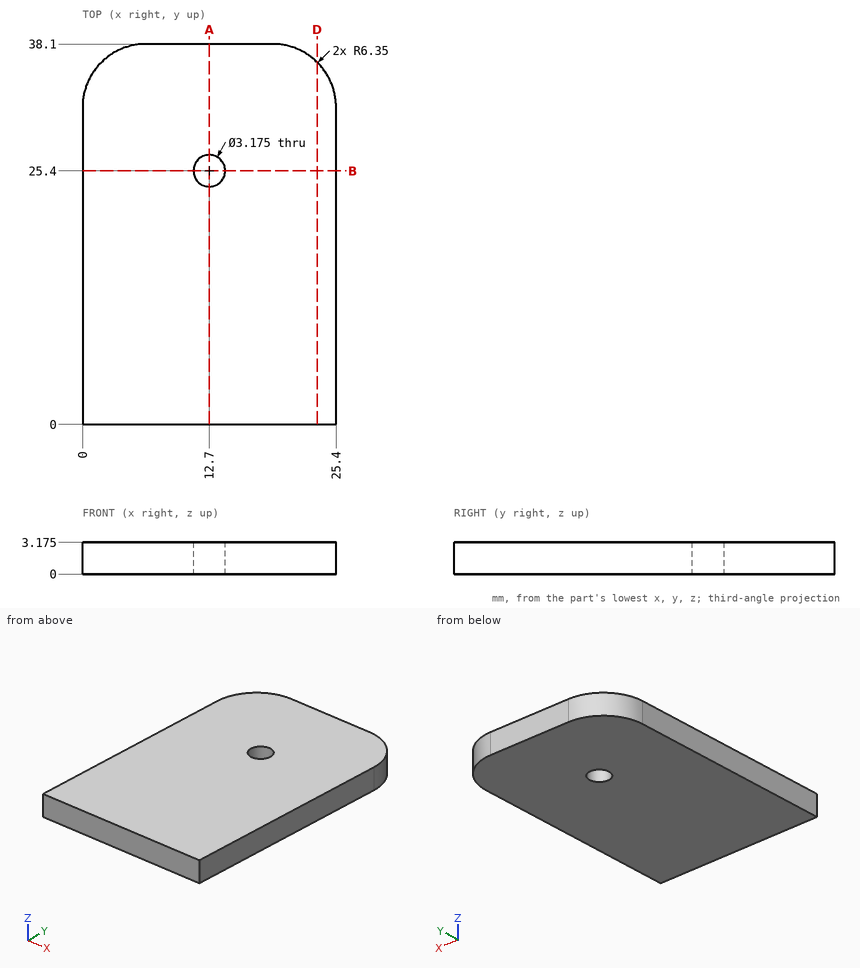
Verification items for this drawing (mm, ordinates from the low corner). Coordinates: 2 decimals unless noted, no trailing zeros. Order: outer loops, then holes, each group sorted by start corner. A loop starts at its lowest first (then second) coordinate and runs counter-clockwise, first axis right, second up. Notation, with made-up numbers: (58.25, -35) - (75.25, -35) arc R21 ccw to (75.25, -26) - close; hole circle Ø5 at (35.25, 70.5). An arc over 180 degrees is marked (long way). Answer in a Markdown table with one row per item. Add a question column.
1. Section check D-D (x = 23.5). Enter the section's corners in (y, z) (3 decimals), plus the area to 3 significant figures.
2. Section check A-A (x = 12.7). Enter the section's corners in (y, z) (1 decimal), plus the area to 3 significant figures.
3. Material ranges on L1, parallel to Y at x = 12.7, z = 1.7; L2, parallel to X at y = 25, z = 2.2; L3, parallel to Y at x = 14, z = 1.3, recorded low to high. Write a range as [from, to].
4. Section check B-B (y = 25.4). Enter the section's corners in (x, z) (1 decimal).
Data:
| question | item | result |
|---|---|---|
| 1 | outline | (0, 0) - (36.28, 0) - (36.28, 3.175) - (0, 3.175) - close |
| 1 | area | 115 mm² |
| 2 | outline | (0, 0) - (23.8, 0) - (23.8, 3.2) - (0, 3.2) - close; (27, 0) - (38.1, 0) - (38.1, 3.2) - (27, 3.2) - close |
| 2 | area | 111 mm² |
| 3 | L1 | y = [0, 23.81], [26.99, 38.1] |
| 3 | L2 | x = [0, 11.16], [14.24, 25.4] |
| 3 | L3 | y = [0, 24.49], [26.31, 38.1] |
| 4 | outline | (0, 0) - (11.1, 0) - (11.1, 3.2) - (0, 3.2) - close; (14.3, 0) - (25.4, 0) - (25.4, 3.2) - (14.3, 3.2) - close |
